from build123d import *

# Parameters (mm, degrees)
F2_R = 1
F4_D = 5.1


with BuildPart() as f1:
    # F0 (on Front) → F1 (revolve)
    with BuildSketch(Plane.XZ):
        Polygon((-10.2, 61.3408794351), (-13.2, 61.3408794351), (-13.2, 11.3408794351), (-8, -3.6591205649), (-8, -8.6591205649), (0, -8.6591205649), (0, 5.3408794351), (-5.8538794215, 5.3408794351), (-7.4, 11.3408794351), (-10.2, 11.3408794351), align=None)
    revolve(axis=Axis((0, 0, 2.0173949058), (0, 0, -1)))

    # F2
    f2_edges = [f1.edges().sort_by_distance(p)[0] for p in [
        (13.2, 0, 61.340879),
        (10.2, 0, 61.340879),
    ]]
    fillet(f2_edges, radius=F2_R)

    # F4 (through all)
    with Locations(Plane(origin=(0, 0, -8.6591205649), x_dir=(1, 0, 0), z_dir=(0, 0, -1))):
        with Locations((0, 0)):
            Hole(F4_D / 2)


solid = f1.part
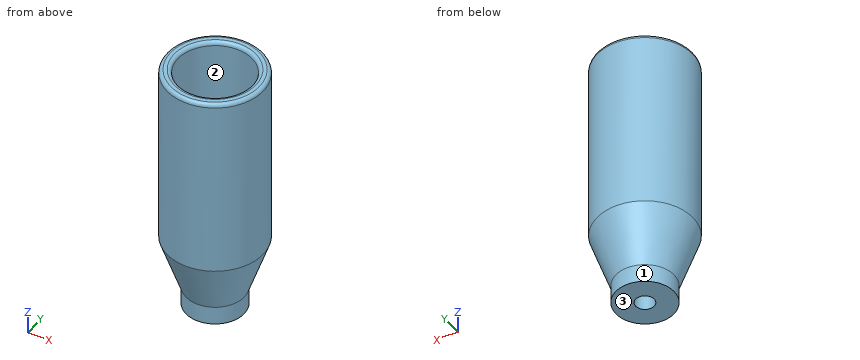
Design review of the part built by this model. Coordinates are the model's own, in mm. Face numbers are marked on the shaded views. Round coordinates to 2 decimals unless told otherwise and drop trailing zeros. Write each loop counter-clockwise with the first axis right and the second up, starting at its lowest first coordinate (ties: lowest second). Pieces come first, ordered by that corner, then holes.
Item 1: Consider section A-A on y = 0. Give the boundary of the cut face in (x, z), and give its area (3 significant figures).
Item 2: For pin 1 Ø8 at (y, z) = (9, 38) entering from +X; pin 2 Ø12 at (y, z) = (9, 23.5) entering from -X; pin 3 Ø8 at (x, y) = (0, 0) entering from +Z; pin 4 Ø2 at (y, z) = (-1, 11) entering from -X, all flat-tipped, find the tip position at first contact; note any pin that passes through.
Item 3: Draft analysis for pull direction Y (two halves, no side actions). For the marked faces 1, 2 and 3, state which applies: released by +Y, released by -Y, zero draft, split by the parting line, or undercut.
Item 4: Wall thickness on L1, parallel to Y at x = 0, z = 39.5; L2, parallel to Z at x = -4, y = -1.5; L3, parallel to X at y = -1.75, z = 46: over which ranges is each line inside the solid? List them lowest first.
Item 5: Consider section C-C on z = 19. Give the boundary of the cut face in (x, y), and give its area (3 significant figures).
Item 6: Consider section D-D on z = 4. Give the boundary of the cut face in (x, y).
Check values:
1. outline: (-13.2, 11.34) - (-8, -3.66) - (-8, -8.66) - (-2.55, -8.66) - (-2.55, 5.34) - (-5.85, 5.34) - (-7.4, 11.34) - (-10.2, 11.34) - (-10.2, 60.34) arc R1 ccw to (-11.2, 61.34) - (-12.2, 61.34) arc R1 ccw to (-13.2, 60.34) - close; (2.55, -8.66) - (8, -8.66) - (8, -3.66) - (13.2, 11.34) - (13.2, 60.34) arc R1 ccw to (12.2, 61.34) - (11.2, 61.34) arc R1 ccw to (10.2, 60.34) - (10.2, 11.34) - (7.4, 11.34) - (5.85, 5.34) - (2.55, 5.34) - close
1. area: 546 mm2
2. pin 1: stops at x = 12.22
2. pin 2: stops at x = -12.85
2. pin 3: stops at z = 5.34
2. pin 4: stops at x = -13.2
3. face 1: split by the parting line
3. face 2: undercut
3. face 3: zero draft
4. L1: y = -13.2 to -10.2, 10.2 to 13.2
4. L2: z = -8.66 to 5.34
4. L3: x = -13.08 to -10.05, 10.05 to 13.08
5. outline: circle Ø26.4 at (0, 0); hole circle Ø20.4 at (0, 0)
5. area: 221 mm2
6. outline: circle Ø21.31 at (0, 0); hole circle Ø5.1 at (0, 0)
